Build history of the part. All positions in model axes, mm. Coordinates: 2 decimals unless noted, no trailing zeros. Order: outer loops, then holes, each group sorted by start corner. A loop starts at its lowest first (then second) coordinate and runs counter-clockwise, first axis right, second up. Notation, with made-up numbers: M -20.75,87 L 27.25,87 A27 cw 27.25,116 Z; hole C -11,-11.75 d3. An arc over 180 degrees is marked long. Write item = value, one per line. Start each with the question number.
Q1. Pin check, flat tips, straight feed: P1, Ø1.5, axis at x = 260, z = 124, coming from the -Y side; P2, Ø4, axis at x = 214, z = 472.5, coming from the +Y side. Stop position of each tip, or through.
Q2. Band-saw the part on C-C on y = -64.5. Write the cut outline in (x, z), plus the area to 3 significant figures.
Q3. Band-saw the part on B-B on x = 280.5. Write the cut outline in (y, z), plus the area to 3 significant figures.
Q4. Pull direction Y, two halves, no side cores. Call faces 1 (the face through (-17.824, -10.554, 394.82)), 2 (the face through (373.11, -114.77, 394.4)), 3 (the face through (-4, -14, 30)): released by +Y, released by -Y, zero draft, split by the parting line, or undercut.
Q5. Drill centre lines: probe 1 along Y at (x, z) = (325.5, 60.5); probe 2 along Y at (x, z) = (174, 658). Where is each one in solid material? Low to high.
Q6. Band-saw the part on A-A on z = 442. Write the cut outline in (x, y), plus the area to 3 significant figures.
```python
from build123d import *

# Parameters (mm, degrees)
AUFSATZ_LINEAR_AUSTRAGEN1_DEPTH = 800
SKIZZE3_R                       = 14.488887394
AUFSATZ_LINEAR_AUSTRAGEN2_DEPTH = 800
SKIZZE5_R                       = 14.488887394
SCHNITT_LINEAR_AUSTRAGEN1_DEPTH = 30
LINEARES_MUSTER1_COUNT          = 2
LINEARES_MUSTER1_PITCH          = 770


with BuildPart() as part:
    # Skizze1 → Aufsatz-Linear austragen1 (new body)
    with BuildSketch(Plane.XY):
        Polygon((0, 0), (383.588464136, -102.782219191), (362.338095958, -127.088200199), (0, -30), (-7.5, -27.990381057), align=None)
    extrude(amount=AUFSATZ_LINEAR_AUSTRAGEN1_DEPTH)

    # Skizze3 → Aufsatz-Linear austragen2 (add)
    with BuildSketch(Plane(origin=(0, 0, 0), x_dir=(-1, 0, 0), z_dir=(0, 0, -1))):
        with Locations((3.75, -13.995190528)):
            Circle(SKIZZE3_R)
    extrude(amount=-AUFSATZ_LINEAR_AUSTRAGEN2_DEPTH)

    # Skizze5 → Schnitt-Linear austragen1 (cut)
    with BuildSketch(Plane(origin=(0, 0, 0), x_dir=(-1, 0, 0), z_dir=(0, 0, -1))):
        with Locations((3.75, -13.995190528)):
            Circle(SKIZZE5_R)
    schnitt_linear_austragen1 = extrude(amount=-SCHNITT_LINEAR_AUSTRAGEN1_DEPTH, mode=Mode.SUBTRACT)

    # Lineares Muster1: Schnitt-Linear austragen1 ×2
    with Locations(*[(0, 0, i * LINEARES_MUSTER1_PITCH) for i in range(1, LINEARES_MUSTER1_COUNT)]):
        add(schnitt_linear_austragen1, mode=Mode.SUBTRACT)


solid = part.part
```
Recorded:
q1.P1 = -99.87
q1.P2 = -56.81
q2.outline = M 128.76,0 L 240.72,0 L 240.72,800 L 128.76,800 Z
q2.area = 89,600 mm2
q3.outline = M -105.16,0 L -75.16,0 L -75.16,800 L -105.16,800 Z
q3.area = 24,000 mm2
q4.face_1 = split by the parting line
q4.face_2 = released by -Y
q4.face_3 = undercut
q5.probe_1 = -117.22 to -87.22
q5.probe_2 = -76.62 to -46.62
q6.outline = M -7.5,-27.99 L 362.34,-127.09 L 383.59,-102.78 L 0,0 A14.49 ccw Z
q6.area = 11,600 mm2
